Check sheet for the modelled part. Datum: model origin and axes. Units: mm. A direction names the side the tool comes from. Round coordinates to 2 decimals unless told otherwise and drop trailing zeros. Write each loop counter-clockwise with the first axis right and the second up, starting at its lowest first coordinate (ties: lowest second). Pieces come first, ordered by that corner, then holes. Notation, with made-up numbers: (29, -12) - (33, -12) arc R23 ccw to (33, 25) - close; hole circle Ø2 at (-33, 39.5). An arc over 180 degrees is marked (long way). Answer as a JSON object with one key per item and string values. Group by question number.
Item 1: Thickness scan on line 1 (Z direction, x = -1.5, y = -9); line 2 (Z direction, x = -2.75, y = 39); line 3 (Y direction, x = -1.55, z = 0). Record the ranges inside material, lowest first.
Item 2: Sectioned sample at C-C on z = 8.25. Record the boundary of the cut face in (x, y).
Item 3: Release check for a two-part mould opening along Z. For faces 1 (the flat face through (3, -2, 7)), 2 (the flat face through (2.56, 17.468, 7.535)), 3 (the flat face through (-3.356, -14, 0)), 4 (the flat face through (3, 5, -10)) record: pulls with the +Z half, pulls with the -Z half, needs draft (parallel to the pull), parting line crosses it, or undercut.
Item 4: Set-up check for faces 5 (the flat face through (3, 36, 5)), 6 (the flat face through (1.4, -2.4, 1.5)), 7 (the flat face through (3, 36, -5)), 8 (the flat face through (0, -23, 0)), 9 (the flat face through (3.356, -1, 0)): record each of +Z, -Z, +X, -X, +Y, -Y from which the full face is reachable in a straight line by a thin tool's end or side.
Item 5: Sectioned sample at B-B on x = 0.75. Record the boundary of the cut face in (y, z).
Item 6: Gauge pin test, flat ends, axial feed: P1, Ø1, axis at y = -12.5, z = -0.5, coming from the +X side; P2, Ø8, axis at y = -9, z = -8, coming from the +X side; P3, Ø2, axis at x = 4.5, y = 23, coming from the -Z side; P4, Ø4.5, axis at y = -5, z = 0, coming from the +X side. Record the tip position at first contact, or that the pin passes through.
Item 7: Sectioned sample at A-A on y = -13. Record the boundary of the cut face in (x, z) (1 decimal).
```python
from build123d import *

# Parameters (mm, degrees)
BOSS_EXTRUDE1_DEPTH = 23
SKETCH2_R           = 2
CUT_EXTRUDE1_DEPTH  = 10
CUT_EXTRUDE2_DEPTH  = 4
BOSS_EXTRUDE2_DEPTH = 5
BOSS_EXTRUDE3_DEPTH = 12


with BuildPart() as part:
    # Sketch1 → Boss-Extrude1 (new body)
    with BuildSketch(Plane(origin=(0, 0, 0), x_dir=(1, 0, 0), z_dir=(0, 1, 0))):
        Polygon((0, -3.875), (3.35584844, -1.9375), (3.35584844, 1.9375), (0, 3.875), (-3.35584844, 1.9375), (-3.35584844, -1.9375), align=None)
    extrude(amount=-BOSS_EXTRUDE1_DEPTH)

    # Sketch2 → Cut-Extrude1 (cut)
    with BuildSketch(Plane.ZY.offset(3.35584844)):
        with Locations(Location((0, -5, 0), (0, 0, 14.361511563))):
            Circle(SKETCH2_R)
    extrude(amount=-CUT_EXTRUDE1_DEPTH, mode=Mode.SUBTRACT)

    # Sketch3 → Cut-Extrude2 (cut)
    with BuildSketch(Plane(origin=(3.35584844, 0, 0), x_dir=(0, 0, -1), z_dir=(1, 0, 0))):
        Polygon((0, -8.464101615), (3, -6.732050808), (3, -3.267949192), (0, -1.535898385), (-3, -3.267949192), (-3, -6.732050808), align=None)
    extrude(amount=-CUT_EXTRUDE2_DEPTH, mode=Mode.SUBTRACT)

    # Sketch4 → Boss-Extrude2 (add, symmetric)
    with BuildSketch(Plane.XY):
        Polygon((-3.35584844, 0), (-3.35584844, 50), (8.64415156, 60.606601718), (8.64415156, 0), align=None)
    extrude(amount=BOSS_EXTRUDE2_DEPTH, both=True)

    # Sketch5 → Boss-Extrude3 (add)
    with BuildSketch(Plane.ZY.offset(3.35584844)):
        Polygon((5, 0), (10, -5), (10, 15.003286349), (5, 20.003286349), align=None)
        Polygon((-10, 15.003286349), (-5, 20.003286349), (-5, 0), (-10, -5), align=None)
    extrude(amount=-BOSS_EXTRUDE3_DEPTH)


solid = part.part
```
Completed:
{
 "1": {"line 1": "-3.01 to 3.01", "line 2": "-5 to 5", "line 3": "-23 to -7, -3 to 51.6"},
 "2": {"outline": "(-3.36, -3.25) - (8.64, -3.25) - (8.64, 16.75) - (-3.36, 16.75) - close"},
 "3": {"face 1": "undercut", "face 2": "pulls with the +Z half", "face 3": "needs draft", "face 4": "pulls with the -Z half"},
 "4": {"face 5": "+Z, +X, -X, +Y", "face 6": "+X", "face 7": "-Z, +X, -X, +Y", "face 8": "+Z, -Z, +X, -X, -Y", "face 9": "+X, -Y"},
 "5": {"outline": "(-23, -3.44) - (0, -3.44) - (0, -5) - (-5, -10) - (15, -10) - (20, -5) - (53.63, -5) - (53.63, 5) - (20, 5) - (15, 10) - (-5, 10) - (0, 5) - (0, 3.44) - (-23, 3.44) - close; hole (-8.46, 0) - (-6.73, -3) - (-3.27, -3) - (-1.54, 0) - (-3.27, 3) - (-6.73, 3) - close"},
 "6": {"P1": "x = 3.36", "P2": "through", "P3": "z = -5", "P4": "x = -0.64"},
 "7": {"outline": "(-3.4, -1.9) - (0, -3.9) - (3.4, -1.9) - (3.4, 1.9) - (0, 3.9) - (-3.4, 1.9) - close"}
}
